The model under review builds one solid part; all positions refer to its coordinate system, in mm. Face numbers are marked on the shaded views. A direction names the side the tool comes from. Give positions to 0.01 mm unless a question says otherwise; leave off trailing zeros. Loops run counter-clockwise (first coordinate to the right, second up) from the corner with the lowest first, then second, coordinate; pieces in that order, holes last. Notation, with made-up numbers: (-28.5, 13.25) - (-19.5, 13.25) arc R29 ccw to (-19.5, 52.25) - close; hole circle Ø9 at (58.5, 79). An arc over 180 degrees is marked (long way). Return JSON: item names as keys, results as strings. Group by question number.
from build123d import *

# Parameters (mm, degrees)
P_IDAT_VYSUNUT_M1_DEPTH  = 10
SKICA2_R                 = 3
ODEBRAT_VYSUNUT_M1_DEPTH = 1
SKICA3_R                 = 2.6
ODEBRAT_VYSUNUT_M2_DEPTH = 7.5
SKICA4_W                 = 23.2
SKICA4_H                 = 1
ODEBRAT_VYSUNUT_M3_DEPTH = 1


with BuildPart() as part:
    # Skica1 → Přidat vysunutím1 (new body)
    with BuildSketch(Plane.XY):
        Polygon((-52.156744291, -7.714704976), (-16.156744291, -7.714704976), (-14.656744291, -6.714704976), (-16.156744291, -5.714704976), (-21.656744291, -5.714704976), (-21.656744291, 1.785295024), (-46.656744291, 1.785295024), (-46.656744291, -5.714704976), (-52.156744291, -5.714704976), (-53.656744291, -6.714704976), align=None)
    extrude(amount=P_IDAT_VYSUNUT_M1_DEPTH)

    # Skica2 → Odebrat vysunutím1 (cut)
    with BuildSketch(Plane(origin=(0, -7.714704976, 0), x_dir=(-1, 0, 0), z_dir=(0, -1, 0))):
        with Locations((43.156744291, -5)):
            Circle(SKICA2_R)
        with Locations((37.146744291, -5)):
            Circle(SKICA2_R)
        with Locations((31.136744291, -5)):
            Circle(SKICA2_R)
        with Locations((25.126744291, -5)):
            Circle(SKICA2_R)
    extrude(amount=-ODEBRAT_VYSUNUT_M1_DEPTH, mode=Mode.SUBTRACT)

    # Skica3 → Odebrat vysunutím2 (cut)
    with BuildSketch(Plane(origin=(0, -6.714704976, 0), x_dir=(-1, 0, 0), z_dir=(0, -1, 0))):
        with Locations((43.156744291, -5)):
            Circle(SKICA3_R)
        with Locations((37.146744291, -5)):
            Circle(SKICA3_R)
        with Locations((31.136744291, -5)):
            Circle(SKICA3_R)
        with Locations((25.126744291, -5)):
            Circle(SKICA3_R)
    extrude(amount=-ODEBRAT_VYSUNUT_M2_DEPTH, mode=Mode.SUBTRACT)

    # Skica4 → Odebrat vysunutím3 (cut)
    with BuildSketch(Plane(origin=(0, 1.785295024, 0), x_dir=(1, 0, 0), z_dir=(0, 1, 0))):
        with Locations((-34.056744291, -5.129927758)):
            Rectangle(SKICA4_W, SKICA4_H)
    extrude(amount=-ODEBRAT_VYSUNUT_M3_DEPTH, mode=Mode.SUBTRACT)


solid = part.part
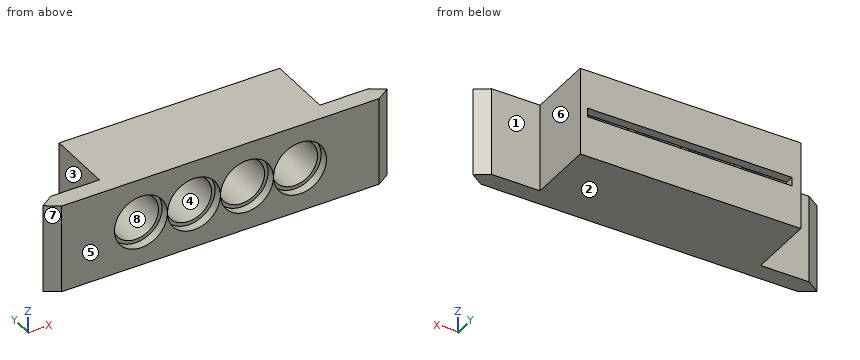
Item 1: For L1, parallel to X at y = -1, z = 5; L2, parallel to Z at x = -41.5, y = 1; L3, parallel to X at y = -6.5, z = 6.25, list the stretches that pass through material, from the lowest coordinate up. Write a range as from..to.
Item 2: Tool access review of the marked faces 1, 2, 3 and 4: name each direction out of +Z, -Z, +X, -X, +Y, -Y from which nothing blocks a thin tool from reaching the whole face with its end or side.
Item 3: Mouldability with a two-part tool opening along X and no side actions: class the marked faces 5, 6, 7 and 8 as +X half, -X half, draft (parallel to the pull), parting line (faces both ways), or undercut.
Item 4: Take a section at A-A (x = -26.5). State the section outline as (y, z) points, then the cut area to 3 significant figures.
Item 5: For P1, Ø2, axis at y = 0.5, z = 2, coming from the +X side; P2, Ø3, axis at y = -5, z = 5, coming from the -X side; P3, Ø1.8, axis at x = -24, z = 3.5, coming from the -Y side, all flat-tipped, find the tip position at first contact; note any pin that passes through.
Item 6: Take a section at B-B (z = 8.5). State the section outline as (x, y) points.
Item 7: Take a section at D-D (z = 5). State how many separate pieces and enclosed holes the cut face has, then the cut area to 3 significant figures.
Item 8: Take a section at C-C (y = -1.25). State the section outline as (x, z) points.
Check sheet entries:
{
 "1": {"L1": "x = -46.66..-45.76, -40.56..-39.75, -34.55..-33.74, -28.54..-27.73, -22.53..-21.66", "L2": "z = 0..4.63, 5.63..10", "L3": "x = -53.33..-45.44, -40.88..-39.43, -34.87..-33.42, -28.86..-27.41, -22.85..-14.98"},
 "2": {"face 1": "+Z, -Z, +X, +Y", "face 2": "-Z, +X, -X, +Y, -Y", "face 3": "+Z, -Z, -X, +Y", "face 4": "-Y"},
 "3": {"face 5": "draft", "face 6": "+X half", "face 7": "-X half", "face 8": "undercut"},
 "4": {"outline": "(-7.71, 0) - (1.79, 0) - (1.79, 4.63) - (0.79, 4.63) - (0.79, 2.79) - (-6.71, 2.79) - (-6.71, 2.33) - (-7.71, 2.33) - close; (-7.71, 7.67) - (-6.71, 7.67) - (-6.71, 7.21) - (0.79, 7.21) - (0.79, 5.63) - (1.79, 5.63) - (1.79, 10) - (-7.71, 10) - close", "area": "55.5 mm^2"},
 "5": {"P1": "stops at x = -21.66", "P2": "stops at x = -53.33", "P3": "stops at y = -6.71"},
 "6": {"outline": "(-53.66, -6.71) - (-52.16, -7.71) - (-16.16, -7.71) - (-14.66, -6.71) - (-16.16, -5.71) - (-21.66, -5.71) - (-21.66, 1.79) - (-46.66, 1.79) - (-46.66, -5.71) - (-52.16, -5.71) - close"},
 "7": {"separate pieces": "5", "enclosed holes": "0", "area": "59.3 mm^2"},
 "8": {"outline": "(-46.66, 0) - (-21.66, 0) - (-21.66, 10) - (-46.66, 10) - close; hole circle Ø5.2 at (-43.16, 5); hole circle Ø5.2 at (-37.15, 5); hole circle Ø5.2 at (-31.14, 5); hole circle Ø5.2 at (-25.13, 5)"}
}
